CAD build for the part. Positions are in the model's coordinates, mm. A direction names the side the tool comes from. Give positions to 0.01 mm unless a question says otherwise; leave off trailing zeros. Loops run counter-clockwise (first coordinate to the right, second up) from the corner with the lowest first, then second, coordinate; pieces in that order, holes last.
Item 1: Mould opens along X. For faces 4 (the flat face through (-45.042, -20, 40)), 5 (the flat face through (-109.042, -28, 40)), 6 (the flat face through (-111.042, -20, 40)) say: released by +X, released by -X, zero draft, split by the parting line, or undercut.
Item 2: Saw through at B-B on y = -28. Give the cut face in (x, z), plus the area to 3 significant figures.
Item 3: Saw through at C-C on x = -74.5. Give the cut face in (y, z), plus the area to 3 significant figures.
Item 4: Saw through at D-D on z = 5. Give the cut face in (x, y).
Item 5: Saw through at A-A on y = -14.5. Give the cut face in (x, z).
Item 6: Drop flat-ended pins along their axis: P1, Ø20, axis at y = -22.5, z = 46, coming from the -X side; P2, Ø1.5, axis at x = -110, y = -24, coming from the +Z side; P3, Ø2.5, axis at x = -47, y = -15, coming from the -Z side. Give the stop position or say it passes through.
Item 7: Which spindle directions (+Z, -Z, +X, -X, +Y, -Y) get a long thin tool onto all of the face, cutting with end or side? Do faces 1 (the flat face through (-48.042, -20, 40)), 2 (the cylindrical face through (-46.563, -29.475, 43.686)), 3 (the cylindrical face through (-108.535, -37.404, 35.238)). Say none if no direction does.
Item 8: Probe probe 1 along X at (y, z) = (-35, 50.5); probe 2 along X at (y, z) = (-25, 36); probe 3 along Z at (x, y) = (-48, -11.5). List the from-to ranges inside material, lowest first.
from build123d import *

# Parameters (mm, degrees)
SKETCH1_W           = 110
SKETCH1_H           = 180
BOSS_EXTRUDE1_DEPTH = 0.5
SKETCH1_3_W         = 3
SKETCH1_3_H         = 25
BOSS_EXTRUDE2_DEPTH = 40
SKETCH3_R           = 10.6
CUT_EXTRUDE1_DEPTH  = 1
SKETCH4_R           = 3.85
CUT_EXTRUDE2_DEPTH  = 161.494936001


with BuildPart() as part:
    # Sketch1 → Boss-Extrude1 (new body)
    with BuildSketch(Plane(origin=(0, 0, 0), x_dir=(1, 0, 0), z_dir=(0, 1, 0))):
        with Locations((-78.042251664, -40.129260668)):
            Rectangle(SKETCH1_W, SKETCH1_H)
    extrude(amount=BOSS_EXTRUDE1_DEPTH)

    # Sketch1<3> → Boss-Extrude2 (add)
    with BuildSketch(Plane(origin=(0, 0, 0), x_dir=(1, 0, 0), z_dir=(0, 1, 0))):
        with Locations((-109.542251664, -40.129260668)):
            Rectangle(SKETCH1_3_W, SKETCH1_3_H)
        with Locations((-46.542251664, -40.129260668)):
            Rectangle(SKETCH1_3_W, SKETCH1_3_H)
    extrude(amount=-BOSS_EXTRUDE2_DEPTH)

    # Sketch3 → Cut-Extrude1 (cut)
    with BuildSketch(Plane(origin=(-108.042251664, 0, 0), x_dir=(0, 0, -1), z_dir=(1, 0, 0))):
        with Locations((-40.129260668, -28)):
            Circle(SKETCH3_R)
    extrude(amount=-CUT_EXTRUDE1_DEPTH, mode=Mode.SUBTRACT)

    # Sketch4 → Cut-Extrude2 (cut, through all)
    with BuildSketch(Plane.ZY.offset(48.042251664)):
        with Locations((40.129260668, -28)):
            Circle(SKETCH4_R)
    extrude(amount=-CUT_EXTRUDE2_DEPTH, mode=Mode.SUBTRACT)


solid = part.part
Results below:
1. face 4: released by +X
1. face 5: undercut
1. face 6: released by -X
2. outline: (-111.04, 27.63) - (-108.04, 27.63) - (-108.04, 29.53) - (-109.04, 29.53) - (-109.04, 50.73) - (-108.04, 50.73) - (-108.04, 52.63) - (-111.04, 52.63) - close; (-48.04, 27.63) - (-45.04, 27.63) - (-45.04, 36.28) - (-48.04, 36.28) - close; (-48.04, 43.98) - (-45.04, 43.98) - (-45.04, 52.63) - (-48.04, 52.63) - close
2. area: 106 mm2
3. outline: (0, -49.87) - (0.5, -49.87) - (0.5, 130.13) - (0, 130.13) - close
3. area: 90.0 mm2
4. outline: (-133.04, 0) - (-23.04, 0) - (-23.04, 0.5) - (-133.04, 0.5) - close
5. outline: (-111.04, 27.63) - (-108.04, 27.63) - (-108.04, 52.63) - (-111.04, 52.63) - close; (-48.04, 27.63) - (-45.04, 27.63) - (-45.04, 52.63) - (-48.04, 52.63) - close
6. P1: stops at x = -111.04
6. P2: stops at z = 52.63
6. P3: stops at z = 27.63
7. face 1: +Z, -Z, -Y
7. face 2: +X
7. face 3: none
8. probe 1: x = -111.04 to -108.04, -48.04 to -45.04
8. probe 2: x = -111.04 to -109.04, -48.04 to -45.04
8. probe 3: z = 27.63 to 52.63
